Geometry check sheet. Reference: the model listing, model coordinates, mm. A direction names the side the tool comes from. Round coordinates to 2 decimals unless told otherwise and drop trailing zeros. Write each loop counter-clockwise with the first axis right and the second up, starting at its lowest first coordinate (ties: lowest second). Pieces come first, ordered by that corner, then holes.
Item 1: Scan lines: probe 1 along Y at (x, z) = (4, -2.25); probe 2 along Z at (x, y) = (11.5, 17.75). Record each from-to range of solid material in increasing order.
Item 2: Cross-section at C-C (z = -3.5). Enter the section's corners in (x, y), then the cut area to 3 significant figures.
Item 3: Cross-section at B-B (y = 9.5). Enter the section's corners in (x, z), then the cut area to 3 significant figures.
Item 4: Depth check by flat-ended pin: P1, Ø1, axis at x = 18.5, y = 8, coming from the -Z side; P2, Ø0.6, axis at x = 5, y = 25, coming from the -Z side. Enter the tip coordinate at first touch or a pass-through.
Item 5: Cross-section at A-A (z = -1.5). Enter the section's corners in (x, y).
Item 6: Access from +Z, -Z, +X, -X, +Y, -Y to the whole of each face (thin tool, end or side, straight path). Record for faces 5 (the face through (0, 13, -2)), 6 (the face through (4, 23.5, -2)), 7 (the face through (1.198, 24.768, -6.068)), 8 (the face through (17.4, 20.9, -4.9)).
Item 7: Cross-section at D-D (x = 8.75). Enter the section's corners in (y, z).
Item 8: Draft check along Y on faces 1 (the face through (26.699, 25.715, 0.76)), 2 (the face through (1, 13, -2)), 3 (the face through (14, 13, 0)), 4 (the face through (19, 20, -10)). Enter one of: pulls with the +Y half, pulls with the -Y half, needs draft (parallel to the pull), parting line crosses it, or undercut.
from build123d import *

# Parameters (mm, degrees)
F0_W     = 27
F0_H     = 26
F1_DEPTH = 1.5
F3_DEPTH = 2.5
F5_DEPTH = 26
F7_R     = 2
F8_DEPTH = 10
F9_R     = 1
F10_R    = 1


# Not quite as in the source:
# - a pattern or mirror of a feature is missing from the dataset's text; its kind, count and spacing are read off the source's solid


with BuildPart() as f1:
    # F0 (on Top) → F1 (new body)
    with BuildSketch(Plane.XY):
        with Locations((13.5, 13)):
            Rectangle(F0_W, F0_H)
    extrude(amount=F1_DEPTH)

    # F2 (on Front) → F3 (join)
    with BuildSketch(Plane.XZ):
        with BuildLine():
            Line((2, 0), (0, 0))
            Line((0, 0), (0, -6.5))
            Line((0, -6.5), (0.8364939141, -6.5))
            Line((0.8364939141, -6.5), (1.5690374528, -5.6242691353))
            ThreePointArc((1.5690374528, -5.6242691353), (1.0835712802, -4.2466571982), (2, -3.1092696409))
            Line((2, -3.1092696409), (2, 0))
        make_face()
        with BuildLine():
            Line((8, 0), (3, 0))
            Line((3, 0), (3, -3.0653657134))
            ThreePointArc((3, -3.0653657134), (3.7676272431, -3.6075221422), (4.0620223023, -4.5))
            ThreePointArc((4.0620223023, -4.5), (3.9294061684, -5.1166533571), (3.5550071518, -5.6242691353))
            Line((3.5550071518, -5.6242691353), (4.1543185927, -6.5))
            Line((4.1543185927, -6.5), (5.2601844187, -6.5))
            Line((5.2601844187, -6.5), (8, 0))
        make_face()
        with BuildLine():
            Line((3, 0), (2, 0))
            Line((2, 0), (2, -3.1092696409))
            ThreePointArc((2, -3.1092696409), (2.4962297898, -3.0014435795), (3, -3.0653657134))
            Line((3, -3.0653657134), (3, 0))
        make_face()
    f3 = extrude(amount=-F3_DEPTH)

    # F3_copies: F3 across plane
    add(f3.mirror(Plane.ZX.offset(13)))

    # F4 (on Front) → F5 (join, through all)
    with BuildSketch(Plane.XZ):
        Polygon((2, 0), (0, 0), (0, -4), align=None)
    extrude(amount=-F5_DEPTH)

    # F7 (on face) → F8 (join)
    with BuildSketch(Plane(origin=(0, 0, 0), x_dir=(1, 0, 0), z_dir=(0, 0, -1))):
        with Locations((19, -19.7)):
            Circle(F7_R)
    extrude(amount=F8_DEPTH)

    # F9
    f9_edges = [f1.edges().sort_by_distance(p)[0] for p in [
        (17, 19.7, 0),
        (17, 19.7, -10),
    ]]
    fillet(f9_edges, radius=F9_R)

    # F10
    f10_edges = [f1.edges().sort_by_distance(p)[0] for p in [
        (27, 26, 0.75),
        (27, 0, 0.75),
    ]]
    fillet(f10_edges, radius=F10_R)


solid = f1.part
Resolved:
1. probe 1: y = 0 to 2.5, 23.5 to 26
1. probe 2: z = 0 to 1.5
2. outline: (0, 0) - (1.44, 0) - (1.44, 2.5) - (0.25, 2.5) - (0.25, 23.5) - (1.44, 23.5) - (1.44, 26) - (0, 26) - close; (3.68, 0) - (6.52, 0) - (6.52, 2.5) - (3.68, 2.5) - close; (3.68, 23.5) - (6.52, 23.5) - (6.52, 26) - (3.68, 26) - close; circle Ø4 at (19, 19.7)
2. area: 39.3 mm2
3. outline: (0, -4) - (2, 0) - (27, 0) - (27, 1.5) - (0, 1.5) - close
3. area: 44.5 mm2
4. P1: stops at z = 0
4. P2: stops at z = -6.5
5. outline: (0, 0) - (7.37, 0) - (7.37, 2.5) - (1.25, 2.5) - (1.25, 23.5) - (7.37, 23.5) - (7.37, 26) - (0, 26) - close; circle Ø4 at (19, 19.7)
6. face 5: +Z, -Z, -X, +Y, -Y
6. face 6: -Z, +X
6. face 7: -Z, +Y, -Y
6. face 8: -Z
7. outline: (0, 0) - (26, 0) - (26, 1.5) - (0, 1.5) - close
8. face 1: pulls with the +Y half
8. face 2: undercut
8. face 3: undercut
8. face 4: needs draft
